```python
from build123d import *

# Parameters (mm, degrees)
BOSS_EXTRUDE1_DEPTH     = 15
CUT_EXTRUDE1_DEPTH      = 45.432533126
CUT_EXTRUDE1_DEPTH_BACK = 45.432533126
SKETCH3_W               = 35.5
SKETCH3_H               = 1.5
BOSS_EXTRUDE2_DEPTH     = 15
BOSS_EXTRUDE3_DEPTH     = 13.5
SKETCH5_W               = 37
SKETCH5_H               = 69.5
BOSS_EXTRUDE4_DEPTH     = 1.5
FILLET1_R               = 8
SKETCH6_R               = 2.5
CUT_EXTRUDE2_DEPTH      = 1.5
FILLET2_R               = 1
CUT_EXTRUDE3_DEPTH      = 61.3158354
CUT_EXTRUDE3_DEPTH_BACK = 61.3158354
SKETCH7_R               = 0.75


with BuildPart() as part:
    # Sketch1 → Boss-Extrude1 (new body)
    with BuildSketch(Plane(origin=(0, 0, 0), x_dir=(1, 0, 0), z_dir=(0, 1, 0))):
        Polygon((17.5, 35.5), (-18, 35.5), (-18, -35.5), (17.5, -35.5), (17.5, -37), (-19.5, -37), (-19.5, 37), (17.5, 37), align=None)
    extrude(amount=BOSS_EXTRUDE1_DEPTH)

    # Sketch2 → Cut-Extrude1 (cut, two sides: drawn at the far end of the back side and taken through both)
    with BuildSketch(Plane(origin=(0, 15, 0), x_dir=(1, 0, 0), z_dir=(0, 1, 0)).offset(-CUT_EXTRUDE1_DEPTH_BACK)):
        Polygon((17.5, -35.5), (17.5, -37), (28.422753275, -37), (28.422753275, -32.5), (-18, -32.5), (-18, -35.5), align=None)
        Polygon((-19.5, -32.5), (-19.5, -37), (17.5, -37), (17.5, -35.5), (-18, -35.5), (-18, -32.5), align=None)
    extrude(amount=CUT_EXTRUDE1_DEPTH + CUT_EXTRUDE1_DEPTH_BACK, mode=Mode.SUBTRACT)

    # Sketch3 → Boss-Extrude2 (add)
    with BuildSketch(Plane(origin=(0, 15, 0), x_dir=(1, 0, 0), z_dir=(0, 1, 0))):
        with Locations((-0.25, -31.75)):
            Rectangle(SKETCH3_W, SKETCH3_H)
    extrude(amount=-BOSS_EXTRUDE2_DEPTH)

    # Sketch4 → Boss-Extrude3 (add)
    with BuildSketch(Plane(origin=(0, 15, 0), x_dir=(1, 0, 0), z_dir=(0, 1, 0))):
        Polygon((-19.5, -32.5), (17.5, -32.5), (17.5, -31), (-18, -31), (-18, 35.5), (17.5, 35.5), (17.5, 37), (-19.5, 37), align=None)
    extrude(amount=BOSS_EXTRUDE3_DEPTH)

    # Sketch5 → Boss-Extrude4 (add)
    with BuildSketch(Plane(origin=(0, 28.5, 0), x_dir=(1, 0, 0), z_dir=(0, 1, 0))):
        with Locations((-1, 2.25)):
            Rectangle(SKETCH5_W, SKETCH5_H)
    extrude(amount=BOSS_EXTRUDE4_DEPTH)

    # Fillet1
    fillet1_edges = [part.edges().sort_by_distance(p)[0] for p in [
        (-18, 28.5, -2.25),
        (-19.5, 30, -2.25),
    ]]
    fillet(fillet1_edges, radius=FILLET1_R)

    # Sketch6 → Cut-Extrude2 (cut)
    with BuildSketch(Plane.XY.offset(32.5)):
        with BuildLine():
            Line((-5, 15.1), (-16.5, 15.1))
            Line((-16.5, 15.1), (-16.5, 8.53719171))
            Line((-16.5, 8.53719171), (17.5, 8.53719171))
            Line((17.5, 8.53719171), (17.5, 15.1))
            Line((17.5, 15.1), (5, 15.1))
            Line((5, 15.1), (5, 21.1))
            ThreePointArc((5, 21.1), (0, 26.1), (-5, 21.1))
            Line((-5, 21.1), (-5, 15.1))
        make_face()
        with Locations((-11, 21.1)):
            Circle(SKETCH6_R)
        with Locations((11, 21.1)):
            Circle(SKETCH6_R)
    extrude(amount=-CUT_EXTRUDE2_DEPTH, mode=Mode.SUBTRACT)

    # Fillet2
    fillet2_edges = [part.edges().sort_by_distance(p)[0] for p in [
        (5, 15.1, 31.75),
        (17.5, 15.1, 31.75),
        (17.5, 8.53719171, 31.75),
        (-16.5, 8.53719171, 31.75),
        (-16.5, 15.1, 31.75),
        (-5, 15.1, 31.75),
    ]]
    fillet(fillet2_edges, radius=FILLET2_R)

    # Sketch7 → Cut-Extrude3 (cut, two sides: drawn at the far end of the back side and taken through both)
    with BuildSketch(Plane.ZY.offset(19.5).offset(-CUT_EXTRUDE3_DEPTH_BACK)):
        with Locations((25, 1.5)):
            Circle(SKETCH7_R)
        with Locations((0, 1.5)):
            Circle(SKETCH7_R)
        with Locations((-25, 1.5)):
            Circle(SKETCH7_R)
    extrude(amount=CUT_EXTRUDE3_DEPTH + CUT_EXTRUDE3_DEPTH_BACK, mode=Mode.SUBTRACT)


solid = part.part
```
Can you work these out from the model? Positions are in its coordinate system, mm. A direction names the side the tool comes from. Give positions to 0.01 mm unless a question says otherwise; leave off trailing zeros. Loops run counter-clockwise (first coordinate to the right, second up) from the corner with the lowest first, then second, coordinate; pieces in that order, holes last. Notation, with made-up numbers: M 46,7 L 65,7 A36 cw 65,46 Z; hole C 30,51.5 d4. An arc over 180 degrees is marked long. One line per item, written item: value.
(1) Suppose I cut it at A-A on y = 1.5. List the corners of the cut face in (x, z) for me.
Returned:
outline: M -19.5,-37 L 17.5,-37 L 17.5,-35.5 L -18,-35.5 L -18,-25.75 L -19.5,-25.75 Z; M -19.5,-24.25 L -18,-24.25 L -18,-0.75 L -19.5,-0.75 Z; M -19.5,0.75 L -18,0.75 L -18,24.25 L -19.5,24.25 Z; M -19.5,25.75 L -18,25.75 L -18,31 L 17.5,31 L 17.5,32.5 L -19.5,32.5 Z
(2) We'd pull the mould along Y, two halves only. Please class faces 5 (the face through (-18.74, 1.53, 24.25)), 6 (the face through (4, 28.5, -3)), 7 (the face through (0, 8, 31)), 8 (the face through (0, 8.537, 32)): released by +Y, released by -Y, zero draft, split by the parting line, or undercut.
Returned:
face 5: undercut
face 6: released by -Y
face 7: zero draft
face 8: undercut
(3) Which directions (+Z, -Z, +X, -X, +Y, -Y) give clear straight access to the entire face, cutting with the end or side of a thin tool? Please do faces 1 (the face through (11, 15.1, 32)), 2 (the face through (0.1, 26.1, 31.8)), 3 (the face through (-1, 15, -37)), 4 (the face through (0, 14, -35.5)).
Returned:
face 1: +Z, +X
face 2: +Z
face 3: -Z, +X, -X, +Y, -Y
face 4: +X, -Y
(4) Suppose I cut it at D-D on x = -0.5. List the corners of the cut face in (y, z) for me, plus the area to 3 significant figures.
Returned:
outline: M 0,-37 L 30,-37 L 30,32.5 L 26.07,32.5 L 26.07,31 L 28.5,31 L 28.5,-35.5 L 0,-35.5 Z; M 0,31 L 8.54,31 L 8.54,32.5 L 0,32.5 Z
area: 163 mm^2
(5) Suppose I cut it at B-B on z = -25. List the corners of the cut face in (x, y) for me, plus the area to 3 significant figures.
Returned:
outline: M -19.5,0 L -18,0 L -18,0.75 L -19.5,0.75 Z; M -19.5,2.25 L -18,2.25 L -18,20.5 A8 cw -10,28.5 L 17.5,28.5 L 17.5,30 L -11.5,30 A8 ccw -19.5,22 Z
area: 96.0 mm^2
(6) Will these pins go through, and if not, where does the flat tip stop? pin 1 (4 mm diameter, centred on x = 11, y = 21.1, fed in from +Z); pin 2 (1.4 mm diameter, centred on y = 1.5, z = 0, fed in from -X); pin 3 (14 mm diameter, centred on x = -1.5, z = -2.5, fed in from -Y); pin 4 (2 mm diameter, centred on y = 18.5, z = 13, fed in from +X).
Returned:
pin 1: z = -35.5
pin 2: through
pin 3: y = 28.5
pin 4: x = -18
(7) Suppose I cut it at C-C on x = 11. List the corners of the cut face in (y, z) for me, plus the area to 3 significant figures.
Returned:
outline: M 0,-37 L 30,-37 L 30,32.5 L 23.6,32.5 L 23.6,31 L 28.5,31 L 28.5,-35.5 L 0,-35.5 Z; M 0,31 L 8.54,31 L 8.54,32.5 L 0,32.5 Z; M 15.1,31 L 18.6,31 L 18.6,32.5 L 15.1,32.5 Z
area: 172 mm^2
(8) I need wall thicknesses on line 1 (Y direction, x = 11, z = 31.95); line 2 (Z direction, x = -18.65, y = 1.5); line 3 (Z direction, x = -16, y = 7). Which ranges of each line are inside material? Lowest first, please.
Returned:
line 1: 0 to 8.54, 15.1 to 18.6, 23.6 to 30
line 2: -37 to -25.75, -24.25 to -0.75, 0.75 to 24.25, 25.75 to 32.5
line 3: -37 to -35.5, 31 to 32.5
